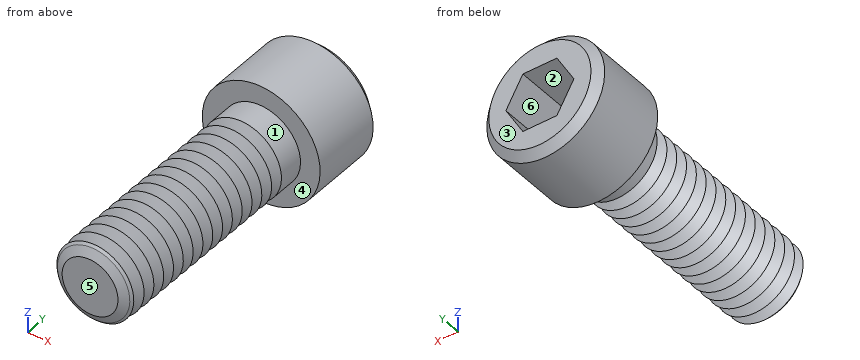
from build123d import *

# Parameters (mm, degrees)
HEX_CUT_DRIVEN_DEPTH = 1.52908


with BuildPart() as part:
    # Sketch3 → Shank Revolve ( driven ) (revolve)
    with BuildSketch(Plane.XY, mode=Mode.PRIVATE) as shank_revolve_driven_sk:
        Polygon((0, 0.65532), (0, -6.35), (0.87376, -6.35), (1.0922, -6.13156), (1.0922, 0.65532), align=None)
    revolve(shank_revolve_driven_sk.sketch.rotate(Axis((0, -50, 0), (0, 1, 0)), 90), axis=Axis((0, -50, 0), (0, 1, 0)))

    # Sketch4 → Thread Revolve Cut ( driven ) (revolve, cut)
    with BuildSketch(Plane.XY, mode=Mode.PRIVATE) as thread_revolve_cut_driven_sk:
        Polygon((0.776909018, -0.889), (1.0922, -0.706966667), (1.633740037, -0.706966667), (1.633740037, -7.260166667), (1.0922, -7.260166667), (0.776909018, -7.078133333), (1.0922, -6.8961), (0.776909018, -6.714066667), (1.0922, -6.532033333), (0.776909018, -6.35), (1.0922, -6.167966667), (0.776909018, -5.985933333), (1.0922, -5.8039), (0.776909018, -5.621866667), (1.0922, -5.439833333), (0.776909018, -5.2578), (1.0922, -5.075766667), (0.776909018, -4.893733333), (1.0922, -4.7117), (0.776909018, -4.529666667), (1.0922, -4.347633333), (0.776909018, -4.1656), (1.0922, -3.983566667), (0.776909018, -3.801533333), (1.0922, -3.6195), (0.776909018, -3.437466667), (1.0922, -3.255433333), (0.776909018, -3.0734), (1.0922, -2.891366667), (0.776909018, -2.709333333), (1.0922, -2.5273), (0.776909018, -2.345266667), (1.0922, -2.163233333), (0.776909018, -1.9812), (1.0922, -1.799166667), (0.776909018, -1.617133333), (1.0922, -1.4351), (0.776909018, -1.253066667), (1.0922, -1.071033333), align=None)
    revolve(thread_revolve_cut_driven_sk.sketch.rotate(Axis((0, -50, 0), (0, 1, 0)), 90), axis=Axis((0, -50, 0), (0, 1, 0)), mode=Mode.SUBTRACT)

    # Sketch5 → Head Revolve ( driven ) (revolve)
    with BuildSketch(Plane.XY, mode=Mode.PRIVATE) as head_revolve_driven_sk:
        Polygon((0, 2.1844), (0, 0), (1.6383, 0), (1.6383, 1.96596), (1.41986, 2.1844), align=None)
    revolve(head_revolve_driven_sk.sketch.rotate(Axis((0, -50, 0), (0, 1, 0)), 90), axis=Axis((0, -50, 0), (0, 1, 0)))

    # Sketch2 → Hex Cut ( driven ) (cut)
    with BuildSketch(Plane(origin=(0, 2.1844, 0), x_dir=(-1, 0, 0), z_dir=(0, 1, 0))):
        Polygon((-0.945872946, 0), (-0.472936473, -0.81915), (0.472936473, -0.81915), (0.945872946, 0), (0.472936473, 0.81915), (-0.472936473, 0.81915), align=None)
    extrude(amount=-HEX_CUT_DRIVEN_DEPTH, mode=Mode.SUBTRACT)


solid = part.part
Design review of the part built by this model. Coordinates are the model's own, in mm. Face numbers are marked on the shaded views. A direction names the side the tool comes from. Round coordinates to 2 decimals unless told otherwise and drop trailing zeros. One line per item, written item: value. Start each with the question number.
1) To check wall thickness, follow L1, parallel to Y at x = -0.15, z = 0.2; L2, parallel to Y at x = -0.3, z = 1.1; L3, parallel to Z at x = 0.2, y = 1.25. State the ranges of each line that lie inside material, in increasing order. Write a range as from..to.
2) For the marked faces 4, 5 and 6, list the 3-axis set-ups (+Z, -Z, +X, -X, +Y, -Y) from which the entire face can be reached by the end or side of a thin tool; tool diameter is ignored.
3) Draft analysis for pull direction Z (two halves, no side actions). For the marked faces 1, 2 and 3, state which applies: +Z half, -Z half, draft (parallel to the pull), parting line (faces both ways), or undercut.
4) Insertion check: pin 1 Ø1 at (y, z) = (-2.5, -0.5) entering from +X; pin 2 Ø1.5 at (x, y) = (1, -0.5) entering from -Z; pin 3 Ø1.5 at (x, y) = (-0.5, -3) entering from +Z. Each pin has a flat end and moves straight along its axis. Give the tip position at first contact, or say it passes through.
Reported:
1. L1: y = -6.35..0.66
1. L2: y = 0..2.18
1. L3: z = -1.63..-0.82, 0.82..1.63
2. face 4: -Y
2. face 5: +Z, -Z, +X, -X, -Y
2. face 6: +Y
3. face 1: parting line
3. face 2: undercut
3. face 3: draft
4. pin 1: stops at x = 1.09
4. pin 2: stops at z = -1.58
4. pin 3: stops at z = 1.09
